Can you work these out from the model? Positions are in its coordinate system, mm. A direction names the side the tool comes from. Give positions to 0.01 mm unless a question says otherwise; leave off trailing zeros. Loops run counter-clockwise (first coordinate to the right, second up) from the corner with the lowest first, then second, coordinate; pieces in that order, holes last. Notation, with made-up numbers: (71, 42.5) -> (89, 42.5) arc R29 cw to (89, 63.5) -> close; hole circle Ø11 at (33.5, 42). An arc over 180 degrees is marked (long way). Use CSV: the item, a comma, the result in double quotes.
Autodesk Inventor part; units mm, degrees
ref_plane "YZ Plane" through (0, 0, 0) normal (1, 0, 0) x (0, 1, 0)
ref_plane "XZ Plane" through (0, 0, 0) normal (0, 1, 0) x (-1, 0, 0)
ref_plane "XY Plane" through (0, 0, 0) normal (0, 0, 1) x (1, 0, 0)
sketch "Sketch1" plane through (0, 0, 0) normal (0, 0, 1) x (1, 0, 0)
  line L0 (-9.525, 16.4978) -> (-28.575, 5.4993)
  arc A0 (-28.575, 5.4993) -> (-28.575, -5.4993) centre (-25.4, 0) ccw
  line L1 (-28.575, -5.4993) -> (-9.525, -16.4978)
  line L2 (9.525, 16.4978) -> (28.575, 5.4993)
  arc A1 (28.575, -5.4993) -> (28.575, 5.4993) centre (25.4, 0) ccw
  line L3 (28.575, -5.4993) -> (9.525, -16.4978)
  arc A2 (-9.525, -16.4978) -> (9.525, -16.4978) centre (0, 0) ccw
  arc A3 (9.525, 16.4978) -> (-9.525, 16.4978) centre (0, 0) ccw
  line L4 (-44.45, 0) -> (44.45, 0) construction
  line L5 (0, -26.67) -> (0, 26.67) construction
  dimension "d0" = 6.35
  dimension "d1" = 50.8
  dimension "d2" = 19.05
extrude "Extrusion1" add sketch "Sketch1" along normal blind 3.175
sketch "Sketch2" plane through (0, 0, 3.175) normal (0, 0, 1) x (1, 0, 0)
  point P0 (0, 0)
hole "Hole1" at (0, 0, 3.175) direction (0, 0, -1) diameter 28.575 end through all counterbore diameter 31.75 counterbore depth 1.5875
sketch "Sketch3" plane through (0, 0, 3.175) normal (0, 0, 1) x (1, 0, 0)
  arc A0 (-28.575, 5.4993) -> (-28.575, -5.4993) centre (-25.4, 0) ccw construction
  arc A1 (28.575, -5.4993) -> (28.575, 5.4993) centre (25.4, 0) ccw construction
  point P0 (0, 0)
  point P1 (-25.4, 0)
hole "Hole2" at (-25.4, 0, 3.175) at (25.4, 0, 3.175) direction (0, 0, -1) diameter 4.9784 end through all
properties part number "Bearing Holder"
(1) If we section it at D-D, the plane x = -24: Write out the boundary of the cut face in (y, z) (3 decimals).
Answer sheet:
outline,"(-8.141, 0) -> (-2.058, 0) -> (-2.058, 3.175) -> (-8.141, 3.175) -> close; (2.058, 0) -> (8.141, 0) -> (8.141, 3.175) -> (2.058, 3.175) -> close"
(2) If we section it at A-A, the plane y = 0: Write out the boundary of the cut face in (x, z) (1 decimal).
Answer sheet:
outline,"(-31.8, 0) -> (-27.9, 0) -> (-27.9, 3.2) -> (-31.8, 3.2) -> close; (-22.9, 0) -> (-14.3, 0) -> (-14.3, 1.6) -> (-15.9, 1.6) -> (-15.9, 3.2) -> (-22.9, 3.2) -> close; (14.3, 0) -> (22.9, 0) -> (22.9, 3.2) -> (15.9, 3.2) -> (15.9, 1.6) -> (14.3, 1.6) -> close; (27.9, 0) -> (31.8, 0) -> (31.8, 3.2) -> (27.9, 3.2) -> close"
(3) If I drill on L1, parallel to Y at x = 0, z = 0.6; L2, parallel to Y at x = 9.5, z = 2.95; L3, parallel to X at y = -8.5, z = 0.6, over which ranges is the centre line in solid material (lowest first)? Write a range as from..to.
Answer sheet:
L1,"y = -19.05..-14.29, 14.29..19.05"
L2,"y = -16.51..-12.72, 12.72..16.51"
L3,"x = -23.38..-11.48, 11.48..23.38"
(4) If we section it at C-C, the plane y = -13: Write out the boundary of the cut face in (x, z) (1 decimal).
Answer sheet:
outline,"(-15.6, 0) -> (-5.9, 0) -> (-5.9, 1.6) -> (-9.1, 1.6) -> (-9.1, 3.2) -> (-15.6, 3.2) -> close; (5.9, 0) -> (15.6, 0) -> (15.6, 3.2) -> (9.1, 3.2) -> (9.1, 1.6) -> (5.9, 1.6) -> close"
(5) If we section it at B-B, the plane x = 0: Write out the boundary of the cut face in (y, z) (1 decimal), then the cut area to 3 significant figures.
Answer sheet:
outline,"(-19.1, 0) -> (-14.3, 0) -> (-14.3, 1.6) -> (-15.9, 1.6) -> (-15.9, 3.2) -> (-19.1, 3.2) -> close; (14.3, 0) -> (19.1, 0) -> (19.1, 3.2) -> (15.9, 3.2) -> (15.9, 1.6) -> (14.3, 1.6) -> close"
area,"25.2 mm2"
(6) Which directions (+Z, -Z, +X, -X, +Y, -Y) give clear straight access to the entire face, cutting with the end or side of a thin tool? Please do faces 1 (the face through (15.497, 3.441, 2.37)), 2 (the face through (27.83, 0.54, 1.57)).
Answer sheet:
face 1,"+Z"
face 2,"+Z, -Z"
(7) We'd pull the mould along Y, two halves only. Please class faces 3 (the face through (0.14, -19.05, 1.57)), 4 (the face through (-0.628, 14.274, 0.783)), 5 (the face through (-27.87, 0.32, 1.57)), 6 (the face through (-15, 0, 0)): released by +Y, released by -Y, zero draft, split by the parting line, or undercut.
Answer sheet:
face 3,"released by -Y"
face 4,"undercut"
face 5,"undercut"
face 6,"zero draft"
(8) Will these pins go through, and if not, where does the flat tip stop? pin 1 Ø1.5 at (x, z) = (7.5, 2.5) entering from +Y; pin 2 Ø1 at (y, z) = (-9, 2.5) entering from -X; pin 3 Ø1 at (x, z) = (-3.5, 1.5) entering from -Y; pin 4 Ø3 at (x, y) = (-25.4, 0) entering from +Z.
Answer sheet:
pin 1,"stops at y = 17.81"
pin 2,"stops at x = -23.38"
pin 3,"stops at y = -18.81"
pin 4,"passes through"
